For this review, use the dimensioned drawing (mm, ordinates from the lowest corner) and the shaded views. Give positions to 0.01 mm unless a question says otherwise; leave off trailing zeros. Order: outer loops, then holes, each group sorted by start corner. A loop starts at its lowest first (then second) coordinate and runs counter-clockwise, first axis right, second up. Notation, with made-up numbers: (76, 12) -> (134, 12) arc R9 cw to (134, 27) -> close; hole circle Ø10 at (-12, 32.5). An arc over 180 degrees is marked (long way). Return JSON: item names as keys, results as strings.
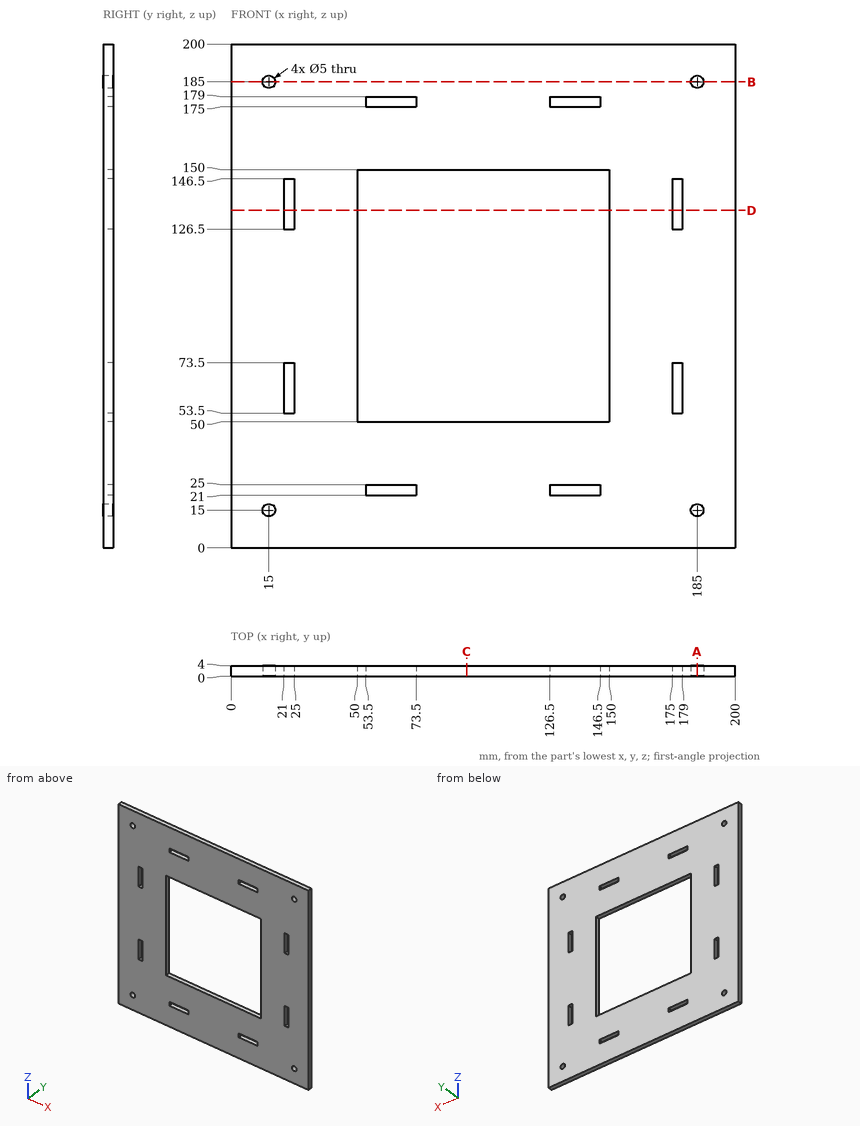
Item 1: Add section B-B (z = 185). Give the boundary of the cut face in (x, y).
Result set:
{"outline": "(0, 0) -> (12.5, 0) -> (12.5, 4) -> (0, 4) -> close; (17.5, 0) -> (182.5, 0) -> (182.5, 4) -> (17.5, 4) -> close; (187.5, 0) -> (200, 0) -> (200, 4) -> (187.5, 4) -> close"}
Item 2: Add section A-A (x = 185). Give the boundary of the cut face in (y, z).
Result set:
{"outline": "(0, 0) -> (4, 0) -> (4, 12.5) -> (0, 12.5) -> close; (0, 17.5) -> (4, 17.5) -> (4, 182.5) -> (0, 182.5) -> close; (0, 187.5) -> (4, 187.5) -> (4, 200) -> (0, 200) -> close"}
Item 3: For pin 1 (1.2 mm diameter, centred on x = 120, y = 3, fed in from -Z); pin 2 (4 mm diameter, centred on x = 15, z = 185, fed in from +Y), all flat-tipped, find the tip position at first contact; note any pin that passes through.
Result set:
{"pin 1": "stops at z = 0", "pin 2": "passes through"}
Item 4: Add section C-C (x = 93.5). Give the boundary of the cut face in (y, z).
Result set:
{"outline": "(0, 0) -> (4, 0) -> (4, 50) -> (0, 50) -> close; (0, 150) -> (4, 150) -> (4, 200) -> (0, 200) -> close"}
Item 5: Add section D-D (z = 134). Give the boundary of the cut face in (x, y).
Result set:
{"outline": "(0, 0) -> (21, 0) -> (21, 4) -> (0, 4) -> close; (25, 0) -> (50, 0) -> (50, 4) -> (25, 4) -> close; (150, 0) -> (175, 0) -> (175, 4) -> (150, 4) -> close; (179, 0) -> (200, 0) -> (200, 4) -> (179, 4) -> close"}
Item 6: Wall thickness on L1, parallel to X at y = 1.75, z = 15; L2, parallel to Z at x = 129, y = 0.85: over which ranges is each line inside the solid? List them lowest first. Write a range as [from, to].
Result set:
{"L1": "x = [0, 12.5], [17.5, 182.5], [187.5, 200]", "L2": "z = [0, 21], [25, 50], [150, 175], [179, 200]"}
